Could you check a few things on this model? Use its own coordinates, in mm. A direction names the side the tool comes from. Round coordinates to 2 decimals unless told otherwise and drop trailing zeros. Loops run counter-clockwise (first coordinate to the right, second up) from the corner with the lowest first, then second, coordinate; pieces in that order, holes last.
from build123d import *

# Parameters (mm, degrees)
F1_DEPTH = 180.34
F3_DEPTH = 32.004
F4_R     = 17.946652
F5_DEPTH = 340.36


with BuildPart() as f1:
    # F0 (on Top) → F1 (new body)
    with BuildSketch(Plane.XY):
        Polygon((76.498292, 35.97128), (-76.308474, 35.97128), (-76.308474, -72.606944), (76.498292, -72.606944), (175.83324, -72.606944), align=None)
    extrude(amount=-F1_DEPTH)

    # F2 (on face) → F3 (join)
    with BuildSketch(Plane(origin=(0, 0, -180.34), x_dir=(1, 0, 0), z_dir=(0, 0, -1))):
        Polygon((-76.308474, -51.736325), (76.498292, -51.736325), (190.256205, 72.606944), (175.83324, 72.606944), (76.498292, -35.97128), (-76.308474, -35.97128), align=None)
    extrude(amount=-F3_DEPTH)

    # F4 (on face) → F5 (cut)
    with BuildSketch(Plane(origin=(-76.308474, 0, 0), x_dir=(0, -1, 0), z_dir=(-1, 0, 0))):
        with Locations((17.826151, -88.319629)):
            Circle(F4_R)
    extrude(amount=-F5_DEPTH, mode=Mode.SUBTRACT)


solid = f1.part
Item 1: If we section it at A-A, the plane y = -4: Please give me the cut outline in (x, z), then the cut area to 3 significant figures.
Results list:
outline: (-76.31, -180.34) - (127.49, -180.34) - (127.49, -148.34) - (113.07, -148.34) - (113.07, -99.76) - (-76.31, -99.76) - close; (-76.31, -76.88) - (113.07, -76.88) - (113.07, 0) - (-76.31, 0) - close
area: 30,300 mm2
Item 2: For faces 1 (the flat face through (56, 40, -148.336)), 2 (the flat face through (59, -72.607, -91)), 3 (the flat face through (1, 35.971, -73)), which set-ups out of +Z, -Z, +X, -X, +Y, -Y let a thin tool reach every point of the face, with its end or its side?
Results list:
face 1: +Z, +X, +Y
face 2: +Z, -Z, +X, -X, -Y
face 3: +Z, +X, -X, +Y
Item 3: If I drill on line 1 along Y through (x, z) = (-20, -119.5); line 2 along Z through (x, y) = (-25, 40); line 3 along Y through (x, z) = (-39, -81), over which ranges is the centre line in solid material (lowest first)?
Results list:
line 1: y = -72.61 to 35.97
line 2: z = -180.34 to -148.34
line 3: y = -72.61 to -34.21, -1.44 to 35.97
Item 4: Will these pins go through, and if not, where does the flat tip stop? pin 1 (4 mm diameter, centred on y = 5.5, z = -128, fed in from +X); pin 2 (10 mm diameter, centred on x = 135.5, y = -9.5, fed in from -Z); pin 3 (2 mm diameter, centred on y = 0.5, z = -88, fed in from +X).
Results list:
pin 1: stops at x = 106.21
pin 2: stops at z = -180.34
pin 3: stops at x = 109.34
Item 5: If we section it at B-B, the plane x = 83.5: Please give me the cut outline in (y, z), then the cut area to 3 significant figures.
Results list:
outline: (-72.61, -180.34) - (44.08, -180.34) - (44.08, -148.34) - (28.32, -148.34) - (28.32, 0) - (-72.61, 0) - close; hole circle Ø35.89 at (-17.83, -88.32)
area: 17,700 mm2
Item 6: If we section it at C-C, the plane z = -143: Please give me the cut outline in (x, y), then the cut area to 3 significant figures.
Results list:
outline: (-76.31, -72.61) - (175.83, -72.61) - (76.5, 35.97) - (-76.31, 35.97) - close
area: 22,000 mm2
Item 7: We'd pull the mould along Z, two halves only. Please class faces 4 (the flat face through (-76.308, -11, -111)), 5 (the cylindrical face through (31.4, -34.4, -95.2)), 6 (the flat face through (25, -11, -180.34)), 7 (the flat face through (20, -18, 0)): released by +Z, released by -Z, zero draft, split by the parting line, or undercut.
Results list:
face 4: zero draft
face 5: undercut
face 6: released by -Z
face 7: released by +Z
Item 8: If we section it at D-D, the plane x = 117.5: Please give me the cut outline in (y, z), then the cut area to 3 significant figures.
Results list:
outline: (-72.61, -180.34) - (6.92, -180.34) - (6.92, -148.34) - (-8.85, -148.34) - (-8.85, -103.86) arc R17.95 cw (long way) to (-8.85, -72.78) - (-8.85, 0) - (-72.61, 0) - close
area: 11,200 mm2
